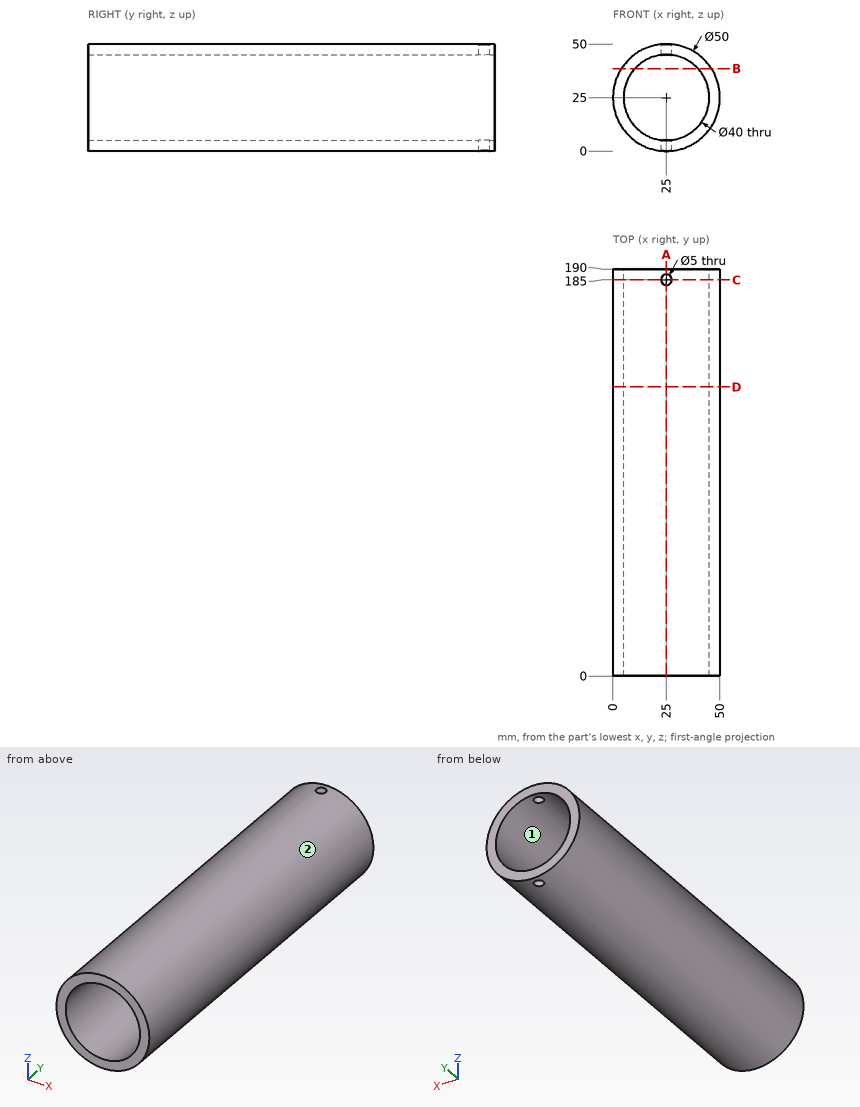
For this review, use the dimensioned drawing (mm, ordinates from the lowest corner) and the shaded views. Coordinates: 2 decimals unless noted, no trailing zeros. Loops run counter-clockwise (first coordinate to the right, second up) from the corner with the lowest first, then second, coordinate; pieces in that order, holes last. Notation, with made-up numbers: (46, -32) -> (93, -32) arc R24 cw to (93, -3) -> close; hole circle Ø9 at (2.5, 68.5). An arc over 180 degrees is marked (long way). Use a Markdown table: item, result. Add a question column.
1. Clearance check with flat-ended pins moving along their axes: pin 1 Ø2 at (x, y) = (19.5, 117.5) entering from -Z; pin 2 Ø10 at (x, y) = (18.5, 57) entering from +Z; pin 3 Ø10 at (y, z) = (143, 14.5) entering from -X. State where each tip first meets the part, or that it passes through.
2. To check wall thickness, follow line 1 (Z direction, x = 25, y = 47.5); line 2 (Y direction, x = 25, z = 3.7); line 3 (Z direction, x = 43, y = 113). State the ranges of each line that lie inside material, in increasing order.
3. Draft analysis for pull direction Z (two halves, no side actions). For the marked faces 1 and 2, state which applies: pulls with the +Z half, pulls with the -Z half, needs draft (parallel to the pull), parting line crosses it, or undercut.
4. Add section B-B on z = 38.5. Write out the cut boundary in (x, y).
5. Add section D-D on y = 135. Write out the cut boundary in (x, z).
6. Add section C-C on y = 185. Write out the cut boundary in (x, z), plus the area to 3 significant figures.
7. Add section A-A on x = 25. Write out the cut boundary in (y, z), plus the area to 3 significant figures.
Returned:
| question | item | result |
|---|---|---|
| 1 | pin 1 | stops at z = 0.41 |
| 1 | pin 2 | stops at z = 49.95 |
| 1 | pin 3 | stops at x = 0.61 |
| 2 | line 1 | z = 0 to 5, 45 to 50 |
| 2 | line 2 | y = 0 to 182.5, 187.5 to 190 |
| 2 | line 3 | z = 7.65 to 16.28, 33.72 to 42.35 |
| 3 | face 1 | undercut |
| 3 | face 2 | parting line crosses it |
| 4 | outline | (3.96, 0) -> (10.24, 0) -> (10.24, 190) -> (3.96, 190) -> close; (39.76, 0) -> (46.04, 0) -> (46.04, 190) -> (39.76, 190) -> close |
| 5 | outline | circle Ø50 at (25, 25); hole circle Ø40 at (25, 25) |
| 6 | outline | (22.5, 0.13) -> (22.5, 5.16) arc R20 cw to (22.5, 44.84) -> (22.5, 49.87) arc R25 ccw to start; (27.5, 0.13) arc R25 ccw to (27.5, 49.87) -> (27.5, 44.84) arc R20 cw to (27.5, 5.16) -> close |
| 6 | area | 657 mm² |
| 7 | outline | (0, 0) -> (182.5, 0) -> (182.5, 5) -> (0, 5) -> close; (0, 45) -> (182.5, 45) -> (182.5, 50) -> (0, 50) -> close; (187.5, 0) -> (190, 0) -> (190, 5) -> (187.5, 5) -> close; (187.5, 45) -> (190, 45) -> (190, 50) -> (187.5, 50) -> close |
| 7 | area | 1,850 mm² |
